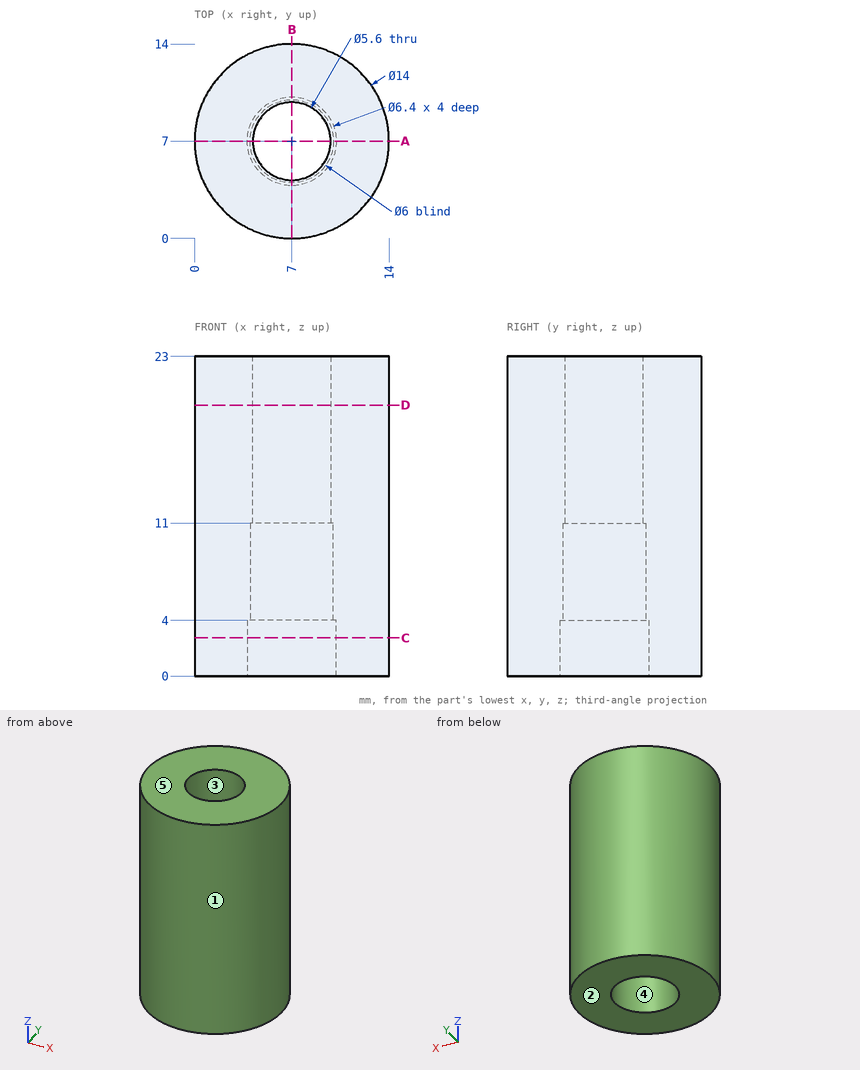
Can you work these out from the drawing? Everything is in mm from the part's minimum corner. A direction names the side the tool comes from. Coordinates: 2 decimals unless noted, no trailing zeros. Write each loop counter-clockwise with the first axis right and the second up, starting at its lowest first coordinate (ties: lowest second). Pieces come first, ordered by that corner, then holes. Notation, with made-up numbers: (9.5, 83.5) -> (48.5, 83.5) arc R28 cw to (48.5, 101.5) -> close; hole circle Ø7 at (30.25, 58). An arc over 180 degrees is marked (long way). Return JSON: item names as keys, results as strings.
(1) I'm going to push flat-ended pins straight in: pin 1 (4 mm diameter, centred on y = 11.5, z = 4, fed in from -X); pin 2 (2 mm diameter, centred on x = 5.5, z = 4.5, fed in from +Y); pin 3 (3 mm diameter, centred on y = 5, z = 18.5, fed in from -X). Where does each tip first touch, or does it pass through?
Numbers:
{"pin 1": "stops at x = 0.46", "pin 2": "stops at y = 13.98", "pin 3": "stops at x = 0.02"}
(2) I need wall thicknesses on L1, parallel to Y at x = 7, z = 1.4; L2, parallel to Y at x = 7, z = 8.75; L3, parallel to X at y = 6.75, z = 5. Which ranges of each line are inside material? Lowest first, please.
Numbers:
{"L1": "y = 0 to 3.8, 10.2 to 14", "L2": "y = 0 to 4, 10 to 14", "L3": "x = 0 to 4.01, 9.99 to 14"}
(3) Imagine slicing it at D-D, the plane z = 19.5. Please give me the cut outline in (x, y).
Numbers:
{"outline": "circle Ø14 at (7, 7); hole circle Ø5.6 at (7, 7)"}
(4) Imagine slicing it at C-C, the plane z = 2.75. Please give me the cut outline in (x, y), then the cut area to 3 significant figures.
Numbers:
{"outline": "circle Ø14 at (7, 7); hole circle Ø6.4 at (7, 7)", "area": "122 mm2"}
(5) We'd pull the mould along X, two halves only. Please class the marked faces 1, 2 and 3: +X half, -X half, draft (parallel to the pull), parting line (faces both ways), or undercut.
Numbers:
{"face 1": "parting line", "face 2": "draft", "face 3": "undercut"}
(6) Imagine slicing it at A-A, the plane y = 7. Please give me the cut outline in (x, z), then the cut area to 3 significant figures.
Numbers:
{"outline": "(0, 0) -> (3.8, 0) -> (3.8, 4) -> (4, 4) -> (4, 11) -> (4.2, 11) -> (4.2, 23) -> (0, 23) -> close; (9.8, 11) -> (10, 11) -> (10, 4) -> (10.2, 4) -> (10.2, 0) -> (14, 0) -> (14, 23) -> (9.8, 23) -> close", "area": "187 mm2"}
(7) Which directions (+Z, -Z, +X, -X, +Y, -Y) give clear straight access to the entire face, cutting with the end or side of a thin tool? Please do the marked faces 4 and 5.
Numbers:
{"face 4": "-Z", "face 5": "+Z, +X, -X, +Y, -Y"}
